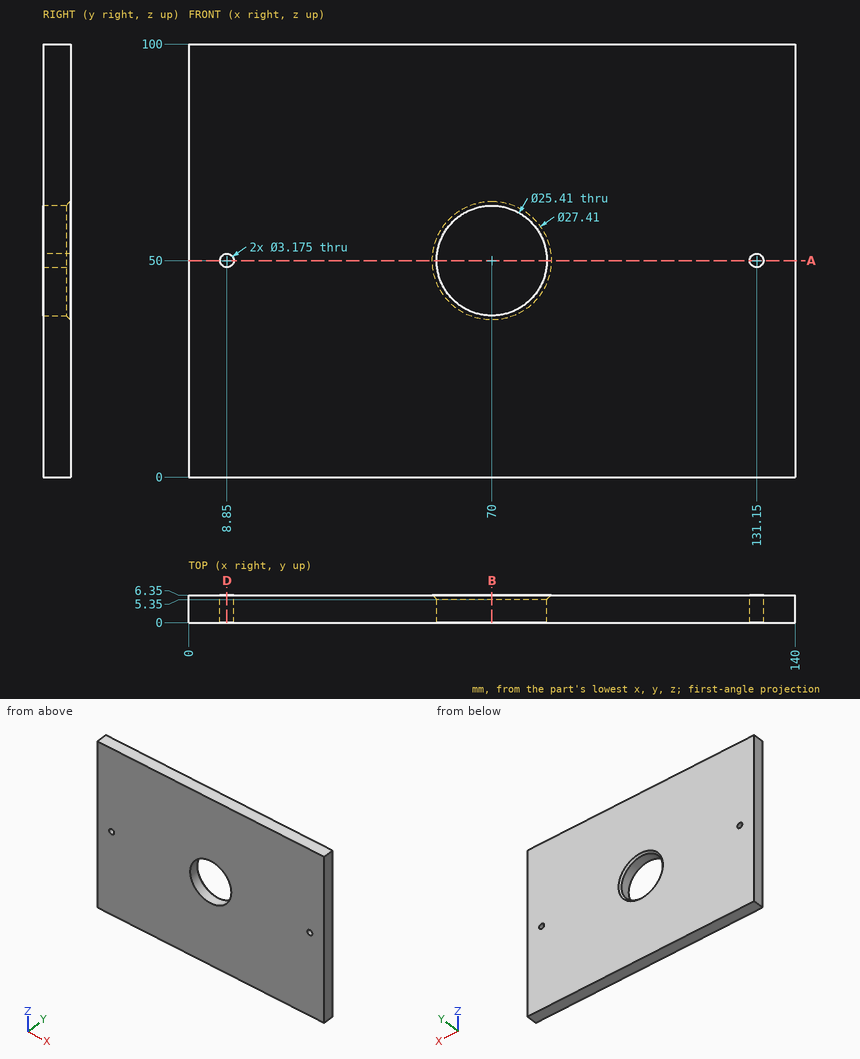
Here's the drawing with two shaded views (mm, measured from the low corner). I have some questions. Round coordinates to 2 decimals unless told otherwise and drop trailing zeros. Order: outer loops, then holes, each group sorted by start corner. A loop starts at its lowest first (then second) coordinate and runs counter-clockwise, first axis right, second up. Notation, with made-up numbers: M 8,-9 L 40,-9 A33 ccw 40,21 Z; hole C -5,38 d3. An arc over 180 degrees is marked long. Use CSV: the item, a comma, the result in double quotes.
1) I need wall thicknesses on line 1 along X through (y, z) = (4.5, 50) (1 decimal); line 2 along Z through (x, y) = (131.15, 2.25); line 3 along X through (y, z) = (0.75, 48). Which ranges of each line are inside material? Lowest first, please. Write a range as [from, to].
Taken from the geometry:
line 1,"[0, 7.3], [10.4, 57.3], [82.7, 129.6], [132.7, 140]"
line 2,"[0, 48.41], [51.59, 100]"
line 3,"[0, 57.45], [82.55, 140]"
2) I want a section at A-A (z = 50). Count the separate pieces of the cut face and the enclosed holes in it, then the cut area to 3 significant figures.
Taken from the geometry:
separate pieces,"4"
enclosed holes,"0"
area,"686 mm^2"
3) I want a section at D-D (x = 8.85). List the corners of the cut face in (y, z) for me, then the cut area to 3 significant figures.
Taken from the geometry:
outline,"M 0,0 L 6.35,0 L 6.35,48.41 L 0,48.41 Z; M 0,51.59 L 6.35,51.59 L 6.35,100 L 0,100 Z"
area,"615 mm^2"
4) I'm going to push a flat-ended pin straight in: P1, Ø3, axis at x = 8.85, z = 50, coming from the +Y side. Where does the tip first touch, or does it pass through?
Taken from the geometry:
P1,"through"
5) I want a section at B-B (x = 70). List the corners of the cut face in (y, z) for me (3 decimals), then the cut area to 3 significant figures.
Taken from the geometry:
outline,"M 0,0 L 6.35,0 L 6.35,36.295 L 5.35,37.295 L 0,37.295 Z; M 0,62.705 L 5.35,62.705 L 6.35,63.705 L 6.35,100 L 0,100 Z"
area,"473 mm^2"
